Work out the finished part from the listing and answer in its coordinate system (mm). Coordinates: 2 decimals unless noted, no trailing zeros. Write each loop counter-clockwise with the first axis right and the second up, starting at its lowest first coordinate (ties: lowest second). Pieces come first, ordered by that corner, then holes. Notation, with made-up numbers: (77.5, 73) - (117.5, 73) arc R16 cw to (117.5, 100) - close; hole circle Ø4 at (89.5, 65). An arc over 180 degrees is marked (long way). Use one line per item in the form item = value. Start each with the question number.
Item 1: A cutting plane is placed at A-A (y = 200). Write down the section's boundary in (x, z).
Item 2: Consider probe 1 along Y at (x, z) = (-10, -1.1); probe 2 along Y at (x, z) = (0, -1.2); probe 3 along Y at (x, z) = (120, -0.85). Determine where each line is inside the solid, lowest interval first.
Item 3: Given pin 1 (21 mm diameter, centred on x = -130, y = 240, fed in from +Z), flat-ended and moving along its own axis, determine where the tip first touches the part or whether it passes through.
Item 4: Determine the mould class of faces 1 (the cylindrical face through (-216.305, 36.887, -0.986)), 2 (the flat face through (-4, 4, -2)) for opening direction X: released by +X, released by -X, zero draft, split by the parting line, or undercut.
from build123d import *

# Parameters (mm, degrees)
SZKIC1_W                   = 550
SZKIC1_H                   = 580
ODGI_CIE_BAZOWE1_DEPTH     = 2
ZAOKR_GLENIE1_R            = 5
WYTNIJ_WYCI_GNI_CIE1_REACH = 401.661
SZKIC2_R                   = 19.6
WYTNIJ_WYCI_GNI_CIE3_REACH = 401.661
SZKIC4_R                   = 2.1
WYTNIJ_WYCI_GNI_CIE4_REACH = 401.661
SZKIC5_R                   = 6.5
WYTNIJ_WYCI_GNI_CIE5_REACH = 401.661
SZKIC6_R                   = 6.5


# Sheet-metal steps are written as plain solids
with BuildPart() as part:
    # Szkic1 → Odgięcie bazowe1 (new body)
    with BuildSketch(Plane.XY):
        Rectangle(SZKIC1_W, SZKIC1_H)
    extrude(amount=-ODGI_CIE_BAZOWE1_DEPTH)

    # Zaokrąglenie1
    zaokr_glenie1_edges = [part.edges().sort_by_distance(p)[0] for p in [
        (275, -290, -1),
        (-275, -290, -1),
    ]]
    fillet(zaokr_glenie1_edges, radius=ZAOKR_GLENIE1_R)

    # Szkic2 → Wytnij-wyciągnięcie1 (cut, up to next)
    with BuildSketch(Plane.XY, mode=Mode.PRIVATE) as wytnij_wyci_gni_cie1_sk1:
        with Locations((-235, 31)):
            Circle(SZKIC2_R)
    wytnij_wyci_gni_cie1_tool1 = extrude(wytnij_wyci_gni_cie1_sk1.sketch, amount=-WYTNIJ_WYCI_GNI_CIE1_REACH, mode=Mode.PRIVATE) & part.part
    # Szkic2 → Wytnij-wyciągnięcie1 (cut, up to next)
    with BuildSketch(Plane.XY, mode=Mode.PRIVATE) as wytnij_wyci_gni_cie1_sk2:
        with Locations((235, 131)):
            Circle(SZKIC2_R)
    wytnij_wyci_gni_cie1_tool2 = extrude(wytnij_wyci_gni_cie1_sk2.sketch, amount=-WYTNIJ_WYCI_GNI_CIE1_REACH, mode=Mode.PRIVATE) & part.part
    add(wytnij_wyci_gni_cie1_tool1.solids().sort_by_distance((-235, 31, 0))[0], mode=Mode.SUBTRACT)
    add(wytnij_wyci_gni_cie1_tool2.solids().sort_by_distance((235, 131, 0))[0], mode=Mode.SUBTRACT)

    # Szkic4 → Wytnij-wyciągnięcie3 (cut, up to next)
    with BuildSketch(Plane.XY, mode=Mode.PRIVATE) as wytnij_wyci_gni_cie3_sk1:
        with Locations((0, 280)):
            Circle(SZKIC4_R)
    wytnij_wyci_gni_cie3_tool1 = extrude(wytnij_wyci_gni_cie3_sk1.sketch, amount=-WYTNIJ_WYCI_GNI_CIE3_REACH, mode=Mode.PRIVATE) & part.part
    # Szkic4 → Wytnij-wyciągnięcie3 (cut, up to next)
    with BuildSketch(Plane.XY, mode=Mode.PRIVATE) as wytnij_wyci_gni_cie3_sk2:
        with Locations((120, 280)):
            Circle(SZKIC4_R)
    wytnij_wyci_gni_cie3_tool2 = extrude(wytnij_wyci_gni_cie3_sk2.sketch, amount=-WYTNIJ_WYCI_GNI_CIE3_REACH, mode=Mode.PRIVATE) & part.part
    # Szkic4 → Wytnij-wyciągnięcie3 (cut, up to next)
    with BuildSketch(Plane.XY, mode=Mode.PRIVATE) as wytnij_wyci_gni_cie3_sk3:
        with Locations((240, 280)):
            Circle(SZKIC4_R)
    wytnij_wyci_gni_cie3_tool3 = extrude(wytnij_wyci_gni_cie3_sk3.sketch, amount=-WYTNIJ_WYCI_GNI_CIE3_REACH, mode=Mode.PRIVATE) & part.part
    # Szkic4 → Wytnij-wyciągnięcie3 (cut, up to next)
    with BuildSketch(Plane.XY, mode=Mode.PRIVATE) as wytnij_wyci_gni_cie3_sk4:
        with Locations(Location((-240, 280, 0), (0, 0, 180))):
            Circle(SZKIC4_R)
    wytnij_wyci_gni_cie3_tool4 = extrude(wytnij_wyci_gni_cie3_sk4.sketch, amount=-WYTNIJ_WYCI_GNI_CIE3_REACH, mode=Mode.PRIVATE) & part.part
    # Szkic4 → Wytnij-wyciągnięcie3 (cut, up to next)
    with BuildSketch(Plane.XY, mode=Mode.PRIVATE) as wytnij_wyci_gni_cie3_sk5:
        with Locations(Location((-120, 280, 0), (0, 0, 180))):
            Circle(SZKIC4_R)
    wytnij_wyci_gni_cie3_tool5 = extrude(wytnij_wyci_gni_cie3_sk5.sketch, amount=-WYTNIJ_WYCI_GNI_CIE3_REACH, mode=Mode.PRIVATE) & part.part
    add(wytnij_wyci_gni_cie3_tool1.solids().sort_by_distance((0, 280, 0))[0], mode=Mode.SUBTRACT)
    add(wytnij_wyci_gni_cie3_tool2.solids().sort_by_distance((120, 280, 0))[0], mode=Mode.SUBTRACT)
    add(wytnij_wyci_gni_cie3_tool3.solids().sort_by_distance((240, 280, 0))[0], mode=Mode.SUBTRACT)
    add(wytnij_wyci_gni_cie3_tool4.solids().sort_by_distance((-240, 280, 0))[0], mode=Mode.SUBTRACT)
    add(wytnij_wyci_gni_cie3_tool5.solids().sort_by_distance((-120, 280, 0))[0], mode=Mode.SUBTRACT)

    # Szkic5 → Wytnij-wyciągnięcie4 (cut, up to next)
    with BuildSketch(Plane(origin=(0, 0, -2), x_dir=(-1, 0, 0), z_dir=(0, 0, -1)), mode=Mode.PRIVATE) as wytnij_wyci_gni_cie4_sk1:
        with Locations((-150, 240)):
            Circle(SZKIC5_R)
    wytnij_wyci_gni_cie4_tool1 = extrude(wytnij_wyci_gni_cie4_sk1.sketch, amount=-WYTNIJ_WYCI_GNI_CIE4_REACH, mode=Mode.PRIVATE) & part.part
    # Szkic5 → Wytnij-wyciągnięcie4 (cut, up to next)
    with BuildSketch(Plane(origin=(0, 0, -2), x_dir=(-1, 0, 0), z_dir=(0, 0, -1)), mode=Mode.PRIVATE) as wytnij_wyci_gni_cie4_sk2:
        with Locations((-130, 240)):
            Circle(SZKIC5_R)
    wytnij_wyci_gni_cie4_tool2 = extrude(wytnij_wyci_gni_cie4_sk2.sketch, amount=-WYTNIJ_WYCI_GNI_CIE4_REACH, mode=Mode.PRIVATE) & part.part
    # Szkic5 → Wytnij-wyciągnięcie4 (cut, up to next)
    with BuildSketch(Plane(origin=(0, 0, -2), x_dir=(-1, 0, 0), z_dir=(0, 0, -1)), mode=Mode.PRIVATE) as wytnij_wyci_gni_cie4_sk3:
        with Locations((-150, 220)):
            Circle(SZKIC5_R)
    wytnij_wyci_gni_cie4_tool3 = extrude(wytnij_wyci_gni_cie4_sk3.sketch, amount=-WYTNIJ_WYCI_GNI_CIE4_REACH, mode=Mode.PRIVATE) & part.part
    # Szkic5 → Wytnij-wyciągnięcie4 (cut, up to next)
    with BuildSketch(Plane(origin=(0, 0, -2), x_dir=(-1, 0, 0), z_dir=(0, 0, -1)), mode=Mode.PRIVATE) as wytnij_wyci_gni_cie4_sk4:
        with Locations((-130, 220)):
            Circle(SZKIC5_R)
    wytnij_wyci_gni_cie4_tool4 = extrude(wytnij_wyci_gni_cie4_sk4.sketch, amount=-WYTNIJ_WYCI_GNI_CIE4_REACH, mode=Mode.PRIVATE) & part.part
    # Szkic5 → Wytnij-wyciągnięcie4 (cut, up to next)
    with BuildSketch(Plane(origin=(0, 0, -2), x_dir=(-1, 0, 0), z_dir=(0, 0, -1)), mode=Mode.PRIVATE) as wytnij_wyci_gni_cie4_sk5:
        with Locations((10, 240)):
            Circle(SZKIC5_R)
    wytnij_wyci_gni_cie4_tool5 = extrude(wytnij_wyci_gni_cie4_sk5.sketch, amount=-WYTNIJ_WYCI_GNI_CIE4_REACH, mode=Mode.PRIVATE) & part.part
    # Szkic5 → Wytnij-wyciągnięcie4 (cut, up to next)
    with BuildSketch(Plane(origin=(0, 0, -2), x_dir=(-1, 0, 0), z_dir=(0, 0, -1)), mode=Mode.PRIVATE) as wytnij_wyci_gni_cie4_sk6:
        with Locations((10, 220)):
            Circle(SZKIC5_R)
    wytnij_wyci_gni_cie4_tool6 = extrude(wytnij_wyci_gni_cie4_sk6.sketch, amount=-WYTNIJ_WYCI_GNI_CIE4_REACH, mode=Mode.PRIVATE) & part.part
    # Szkic5 → Wytnij-wyciągnięcie4 (cut, up to next)
    with BuildSketch(Plane(origin=(0, 0, -2), x_dir=(-1, 0, 0), z_dir=(0, 0, -1)), mode=Mode.PRIVATE) as wytnij_wyci_gni_cie4_sk7:
        with Locations((-10, 220)):
            Circle(SZKIC5_R)
    wytnij_wyci_gni_cie4_tool7 = extrude(wytnij_wyci_gni_cie4_sk7.sketch, amount=-WYTNIJ_WYCI_GNI_CIE4_REACH, mode=Mode.PRIVATE) & part.part
    # Szkic5 → Wytnij-wyciągnięcie4 (cut, up to next)
    with BuildSketch(Plane(origin=(0, 0, -2), x_dir=(-1, 0, 0), z_dir=(0, 0, -1)), mode=Mode.PRIVATE) as wytnij_wyci_gni_cie4_sk8:
        with Locations((130, 220)):
            Circle(SZKIC5_R)
    wytnij_wyci_gni_cie4_tool8 = extrude(wytnij_wyci_gni_cie4_sk8.sketch, amount=-WYTNIJ_WYCI_GNI_CIE4_REACH, mode=Mode.PRIVATE) & part.part
    # Szkic5 → Wytnij-wyciągnięcie4 (cut, up to next)
    with BuildSketch(Plane(origin=(0, 0, -2), x_dir=(-1, 0, 0), z_dir=(0, 0, -1)), mode=Mode.PRIVATE) as wytnij_wyci_gni_cie4_sk9:
        with Locations((150, 220)):
            Circle(SZKIC5_R)
    wytnij_wyci_gni_cie4_tool9 = extrude(wytnij_wyci_gni_cie4_sk9.sketch, amount=-WYTNIJ_WYCI_GNI_CIE4_REACH, mode=Mode.PRIVATE) & part.part
    # Szkic5 → Wytnij-wyciągnięcie4 (cut, up to next)
    with BuildSketch(Plane(origin=(0, 0, -2), x_dir=(-1, 0, 0), z_dir=(0, 0, -1)), mode=Mode.PRIVATE) as wytnij_wyci_gni_cie4_sk10:
        with Locations((150, 240)):
            Circle(SZKIC5_R)
    wytnij_wyci_gni_cie4_tool10 = extrude(wytnij_wyci_gni_cie4_sk10.sketch, amount=-WYTNIJ_WYCI_GNI_CIE4_REACH, mode=Mode.PRIVATE) & part.part
    # Szkic5 → Wytnij-wyciągnięcie4 (cut, up to next)
    with BuildSketch(Plane(origin=(0, 0, -2), x_dir=(-1, 0, 0), z_dir=(0, 0, -1)), mode=Mode.PRIVATE) as wytnij_wyci_gni_cie4_sk11:
        with Locations((130, 240)):
            Circle(SZKIC5_R)
    wytnij_wyci_gni_cie4_tool11 = extrude(wytnij_wyci_gni_cie4_sk11.sketch, amount=-WYTNIJ_WYCI_GNI_CIE4_REACH, mode=Mode.PRIVATE) & part.part
    # Szkic5 → Wytnij-wyciągnięcie4 (cut, up to next)
    with BuildSketch(Plane(origin=(0, 0, -2), x_dir=(-1, 0, 0), z_dir=(0, 0, -1)), mode=Mode.PRIVATE) as wytnij_wyci_gni_cie4_sk12:
        with Locations((-10, 240)):
            Circle(SZKIC5_R)
    wytnij_wyci_gni_cie4_tool12 = extrude(wytnij_wyci_gni_cie4_sk12.sketch, amount=-WYTNIJ_WYCI_GNI_CIE4_REACH, mode=Mode.PRIVATE) & part.part
    add(wytnij_wyci_gni_cie4_tool1.solids().sort_by_distance((150, 240, -2))[0], mode=Mode.SUBTRACT)
    add(wytnij_wyci_gni_cie4_tool2.solids().sort_by_distance((130, 240, -2))[0], mode=Mode.SUBTRACT)
    add(wytnij_wyci_gni_cie4_tool3.solids().sort_by_distance((150, 220, -2))[0], mode=Mode.SUBTRACT)
    add(wytnij_wyci_gni_cie4_tool4.solids().sort_by_distance((130, 220, -2))[0], mode=Mode.SUBTRACT)
    add(wytnij_wyci_gni_cie4_tool5.solids().sort_by_distance((-10, 240, -2))[0], mode=Mode.SUBTRACT)
    add(wytnij_wyci_gni_cie4_tool6.solids().sort_by_distance((-10, 220, -2))[0], mode=Mode.SUBTRACT)
    add(wytnij_wyci_gni_cie4_tool7.solids().sort_by_distance((10, 220, -2))[0], mode=Mode.SUBTRACT)
    add(wytnij_wyci_gni_cie4_tool8.solids().sort_by_distance((-130, 220, -2))[0], mode=Mode.SUBTRACT)
    add(wytnij_wyci_gni_cie4_tool9.solids().sort_by_distance((-150, 220, -2))[0], mode=Mode.SUBTRACT)
    add(wytnij_wyci_gni_cie4_tool10.solids().sort_by_distance((-150, 240, -2))[0], mode=Mode.SUBTRACT)
    add(wytnij_wyci_gni_cie4_tool11.solids().sort_by_distance((-130, 240, -2))[0], mode=Mode.SUBTRACT)
    add(wytnij_wyci_gni_cie4_tool12.solids().sort_by_distance((10, 240, -2))[0], mode=Mode.SUBTRACT)

    # Szkic6 → Wytnij-wyciągnięcie5 (cut, up to next)
    with BuildSketch(Plane(origin=(0, 0, -2), x_dir=(-1, 0, 0), z_dir=(0, 0, -1)), mode=Mode.PRIVATE) as wytnij_wyci_gni_cie5_sk1:
        with Locations((0, 200)):
            Circle(SZKIC6_R)
    wytnij_wyci_gni_cie5_tool1 = extrude(wytnij_wyci_gni_cie5_sk1.sketch, amount=-WYTNIJ_WYCI_GNI_CIE5_REACH, mode=Mode.PRIVATE) & part.part
    # Szkic6 → Wytnij-wyciągnięcie5 (cut, up to next)
    with BuildSketch(Plane(origin=(0, 0, -2), x_dir=(-1, 0, 0), z_dir=(0, 0, -1)), mode=Mode.PRIVATE) as wytnij_wyci_gni_cie5_sk2:
        with Locations((140, 200)):
            Circle(SZKIC6_R)
    wytnij_wyci_gni_cie5_tool2 = extrude(wytnij_wyci_gni_cie5_sk2.sketch, amount=-WYTNIJ_WYCI_GNI_CIE5_REACH, mode=Mode.PRIVATE) & part.part
    # Szkic6 → Wytnij-wyciągnięcie5 (cut, up to next)
    with BuildSketch(Plane(origin=(0, 0, -2), x_dir=(-1, 0, 0), z_dir=(0, 0, -1)), mode=Mode.PRIVATE) as wytnij_wyci_gni_cie5_sk3:
        with Locations((-140, 200)):
            Circle(SZKIC6_R)
    wytnij_wyci_gni_cie5_tool3 = extrude(wytnij_wyci_gni_cie5_sk3.sketch, amount=-WYTNIJ_WYCI_GNI_CIE5_REACH, mode=Mode.PRIVATE) & part.part
    add(wytnij_wyci_gni_cie5_tool1.solids().sort_by_distance((0, 200, -2))[0], mode=Mode.SUBTRACT)
    add(wytnij_wyci_gni_cie5_tool2.solids().sort_by_distance((-140, 200, -2))[0], mode=Mode.SUBTRACT)
    add(wytnij_wyci_gni_cie5_tool3.solids().sort_by_distance((140, 200, -2))[0], mode=Mode.SUBTRACT)


solid = part.part
Answer:
q1.outline = (-275, -2) - (-146.5, -2) - (-146.5, 0) - (-275, 0) - close; (-133.5, -2) - (-6.5, -2) - (-6.5, 0) - (-133.5, 0) - close; (6.5, -2) - (133.5, -2) - (133.5, 0) - (6.5, 0) - close; (146.5, -2) - (275, -2) - (275, 0) - (146.5, 0) - close
q2.probe_1 = -290 to 213.5, 226.5 to 233.5, 246.5 to 290
q2.probe_2 = -290 to 193.5, 206.5 to 277.9, 282.1 to 290
q2.probe_3 = -290 to 277.9, 282.1 to 290
q3.pin_1 = 0
q4.face_1 = undercut
q4.face_2 = zero draft
